Autodesk Inventor part; units mm, degrees
ref_plane "YZ Plane" through (0, 0, 0) normal (1, 0, 0) x (0, 1, 0)
ref_plane "XZ Plane" through (0, 0, 0) normal (0, 1, 0) x (-1, 0, 0)
ref_plane "XY Plane" through (0, 0, 0) normal (0, 0, 1) x (1, 0, 0)
sketch "Sketch1" plane through (0, 0, 0) normal (0, 1, 0) x (-1, 0, 0)
  circle A0 centre (0, 0) radius 25 construction
  line L0 (25, -14.4338) -> (0, -28.8675)
  line L1 (0, -28.8675) -> (-25, -14.4338)
  line L2 (-25, -14.4338) -> (-25, 14.4338)
  line L3 (-25, 14.4338) -> (0, 28.8675)
  line L4 (0, 28.8675) -> (25, 14.4338)
  line L5 (25, 14.4338) -> (25, -14.4338)
  point P0 (25, 0)
  dimension "d0" = 50
extrude "Extrusion1" add sketch "Sketch1" along normal blind 4
properties part number "objeto5"
CAD build for the part. Positions are in the model's coordinates, mm. Give positions to 0.01 mm unless a question says otherwise; leave off trailing zeros. Order: outer loops, then holes, each group sorted by start corner. A loop starts at its lowest first (then second) coordinate and runs counter-clockwise, first axis right, second up.
(1) Saw through at B-B, the plane x = -9. Give the cut face in (y, z), then the cut area to 3 significant figures.
(2) Saw through at C-C, the plane z = 24. Give the cut face in (x, y), then the cut area to 3 significant figures.
(3) Drill centre lines: L1, parallel to X at y = 0.3, z = 22; L2, parallel to Z at x = 20, y = 2.2; L3, parallel to X at y = 0.8, z = 15.5. Where is each one in solid material? Low to high.
(4) Saw through at A-A, the plane y = 3.15. Give the cut face in (x, z).
Results found:
1. outline: (0, -23.67) - (4, -23.67) - (4, 23.67) - (0, 23.67) - close
1. area: 189 mm2
2. outline: (-8.43, 0) - (8.43, 0) - (8.43, 4) - (-8.43, 4) - close
2. area: 67.4 mm2
3. L1: x = -11.89 to 11.89
3. L2: z = -17.32 to 17.32
3. L3: x = -23.15 to 23.15
4. outline: (-25, -14.43) - (0, -28.87) - (25, -14.43) - (25, 14.43) - (0, 28.87) - (-25, 14.43) - close
